Read the model definition and answer for the solid it produces. Units are mm, in the model's axes. Face numbers are marked on the shaded views. Give positions to 0.01 mm unless a question says otherwise; leave off trailing zeros.
Autodesk Inventor part; units mm, degrees
ref_plane "Work Plane1" through (14, 0, 0) normal (1, 0, 0) x (0, 0, -1)
ref_plane "YZ Plane" through (0, 0, 0) normal (1, 0, 0) x (0, 1, 0)
ref_plane "XZ Plane" through (0, 0, 0) normal (0, 1, 0) x (-1, 0, 0)
ref_plane "Work Plane1" through (14, 0, 0) normal (1, 0, 0) x (0, 0, -1)
sketch "Sketch2" plane through (0, 0, 0) normal (1, 0, 0) x (0, 1, 0)
  arc A0 (1.9695, 4.7202) -> (-2.3191, 0.3527) centre (2.9183, -0.5007) ccw
  arc A1 (1.9695, 4.7202) -> (-2.3191, 0.3527) centre (6.9579, -4.4673) ccw
sketch "Sketch5" plane through (14, 0, 0) normal (1, 0, 0) x (0, 0, -1)
  arc A0 (-4.7202, 3.5423) -> (-0.3527, -3.8232) centre (2.3417, 2.7522) ccw
  arc A1 (-4.7202, 3.5423) -> (-0.3527, -3.8232) centre (5.6636, 4.722) ccw
loft "Loft1" add profiles "Sketch2", "Sketch5"
sketch "Sketch7" plane through (0, 0, 0) normal (0, 0, 1) x (1, 0, 0)
  circle A0 centre (0, 0) radius 7.5
  dimension "d10" = 15
extrude "Extrusion3" add sketch "Sketch7" along normal blind 5
pattern_circular "Circular Pattern1" count 7 over 360 about axis through (0, 0, 0) along (0, 0, 1) of "Loft1"
sketch "Sketch8" plane through (0, 0, 5) normal (0, 0, 1) x (1, 0, 0)
  circle A0 centre (0, 0) radius 7.5
  circle A1 centre (0, 0) radius 13.5
  circle A2 centre (0, 0) radius 15
  dimension "d16" = 27
  dimension "d17" = 30
extrude "Extrusion4" cut sketch "Sketch8" against normal blind 5 contours A2
properties part number "fan_3007_blaze"
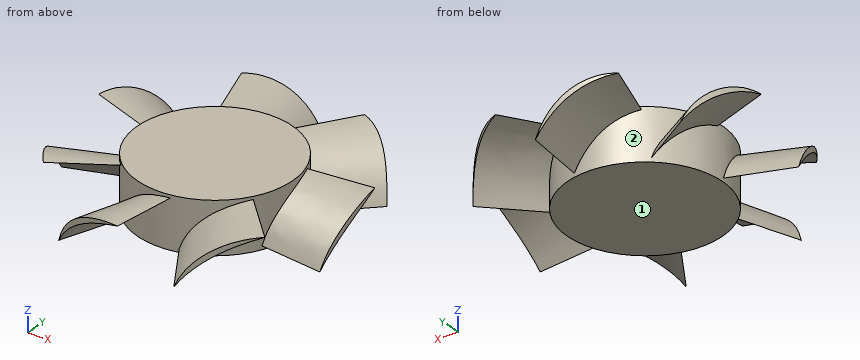
Item 1: Determine the mould class of the marked faces 1 and 2 for opening direction X: pulls with the +X half, pulls with the -X half, needs draft (parallel to the pull), parting line crosses it, or undercut.
Result set:
face 1: needs draft
face 2: undercut
Item 2: Each of these flat-tipped pins is pushed along its axis until it touches: pin 1 Ø3 at (x, z) = (-6.5, 2) entering from +Y; pin 2 Ø2 at (y, z) = (7, 4.5) entering from -X. Where does it stop, or does it pass through?
Result set:
pin 1: stops at y = 7.13
pin 2: stops at x = -12.05
Item 3: Section A-A (x = 10.5) is taken. Give the number of separate pieces and of enclosed holes in the cut face, and give its area (3 significant figures).
Result set:
separate pieces: 3
enclosed holes: 0
area: 3.19 mm2
Item 4: Find the intervals of material crossed by line 1 along Y through (x, z) = (9, 2.9); line 2 along X through (y, z) = (4.25, 1.35); line 3 along Z through (x, y) = (-2, 11.5), in increasing order.
Result set:
line 1: y = -1.68 to -0.92, 8.24 to 9.38
line 2: x = -6.18 to 6.18, 6.45 to 6.88
line 3: z = 3.24 to 3.84
